CAD build for the part. Positions are in the model's coordinates, mm. Give positions to 0.01 mm unless a question says otherwise; leave off trailing zeros. Write each loop counter-clockwise with the first axis right and the second up, starting at its lowest first coordinate (ties: lowest second). Pieces come first, ordered by that corner, then holes. Notation, with made-up numbers: (-14.5, 8.25) - (7.5, 8.25) arc R22 cw to (7.5, 37.25) - close; hole circle Ø10 at (27, 45). An arc over 180 degrees is marked (long way). Answer as a JSON object with one key per item and string values.
from build123d import *

# Parameters (mm, degrees)
F0_W     = 260.35
F0_H     = 260.35
F0_W_2   = 209.55
F0_H_2   = 209.55
F1_DEPTH = 1930.4
F2_W     = 209.55
F2_H     = 330.2
F2_H_2   = 431.8
F2_H_3   = 203.2
F3_DEPTH = 260.35
F4_W     = 209.55
F4_H     = 203.2
F4_H_2   = 431.8
F4_H_3   = 330.2
F5_DEPTH = 260.35


with BuildPart() as f1:
    # F0 (on Top) → F1 (new body)
    with BuildSketch(Plane.XY):
        with Locations((69.85, 69.85)):
            Rectangle(F0_W, F0_H)
        with Locations((69.85, 69.85)):
            Rectangle(F0_W_2, F0_H_2, mode=Mode.SUBTRACT)
    extrude(amount=F1_DEPTH)

    # F2 (on face) → F3 (cut)
    with BuildSketch(Plane.YZ.offset(200.025)):
        with Locations((69.85, 1765.3)):
            Rectangle(F2_W, F2_H)
        with Locations((69.85, 1358.9)):
            Rectangle(F2_W, F2_H_2)
        with Locations((69.85, 901.7)):
            Rectangle(F2_W, F2_H_2)
        with Locations((69.85, 444.5)):
            Rectangle(F2_W, F2_H_2)
        with Locations((69.85, 101.6)):
            Rectangle(F2_W, F2_H_3)
    extrude(amount=-F3_DEPTH, mode=Mode.SUBTRACT)

    # F4 (on face) → F5 (cut)
    with BuildSketch(Plane(origin=(0, 200.025, 0), x_dir=(-1, 0, 0), z_dir=(0, 1, 0))):
        with Locations((-69.85, 101.6)):
            Rectangle(F4_W, F4_H)
        with Locations((-69.85, 444.5)):
            Rectangle(F4_W, F4_H_2)
        with Locations((-69.85, 901.7)):
            Rectangle(F4_W, F4_H_2)
        with Locations((-69.85, 1358.9)):
            Rectangle(F4_W, F4_H_2)
        with Locations((-69.85, 1765.3)):
            Rectangle(F4_W, F4_H_3)
    extrude(amount=-F5_DEPTH, mode=Mode.SUBTRACT)


solid = f1.part
(1) Saw through at B-B, the plane y = 69. State how many separate pieces and enclosed holes the cut face has, and give its area (3 significant figures).
Answer key:
{"separate pieces": "8", "enclosed holes": "0", "area": "5,160 mm²"}
(2) Saw through at A-A, the plane z = 1438.5. Give the cut face in (x, y) (3 decimals).
Answer key:
{"outline": "(-60.325, -60.325) - (-34.925, -60.325) - (-34.925, -34.925) - (-60.325, -34.925) - close; (-60.325, 174.625) - (-34.925, 174.625) - (-34.925, 200.025) - (-60.325, 200.025) - close; (174.625, -60.325) - (200.025, -60.325) - (200.025, -34.925) - (174.625, -34.925) - close; (174.625, 174.625) - (200.025, 174.625) - (200.025, 200.025) - (174.625, 200.025) - close"}
(3) Flat gauge pins, fed straight in: P1, Ø7.5, axis at x = 66, y = -53.5, coming from the +Z side; P2, Ø7.5, axis at x = 95, y = 182.5, coming from the -Z side. Where does each tip first touch, or does it go through?
Answer key:
{"P1": "stops at z = 1600.2", "P2": "stops at z = 203.2"}
(4) Probe L1, parallel to Z at x = 65, y = -40; L2, parallel to Y at x = 182.5, z = 1113 (3 decimals). List the from-to ranges inside material, lowest first. Write a range as [from, to].
Answer key:
{"L1": "z = [203.2, 228.6], [660.4, 685.8], [1117.6, 1143], [1574.8, 1600.2]", "L2": "y = [-60.325, -34.925], [174.625, 200.025]"}
